Read the model definition and answer for the solid it produces. Units are mm, in the model's axes. A direction names the side the tool comes from. Coordinates: 2 decimals unless noted, no trailing zeros. Answer as a JSON object with one key per item and string values. Group by question number.
1) Which of the six approach directions +Z, -Z, +X, -X, +Y, -Y give full straight-line access (tool end or side, diameter ignored) to faces 1 (the face through (-95, -165, -10)), 2 (the face through (-98.068, -167.218, -0.14))?
2) Consider probe 1 along Y at (x, z) = (70, -0.75); probe 2 along Z at (x, y) = (-253, -156.5); probe 3 along Z at (x, y) = (-36, -130). Determine where each line is inside the solid, lowest interval first. Write a range as [from, to].
3) Flat-ended cylindrical pins translate along their axes: P1, Ø1, axis at y = -81.5, z = -0.5, coming from the -X side; P2, Ø10, axis at y = -115.5, z = -2.5, coming from the +X side; P3, Ø3, axis at x = -90.5, z = -2.5, coming from the -Y side. Find the tip coordinate at first contact, or state that the pin passes through.
from build123d import *

# Parameters (mm, degrees)
ESQUISSE4_R             = 1.5
ESQUISSE6_R             = 3
BOSS_EXTRU_1_DEPTH      = 10
ESQUISSE7_R             = 2
ENL_V_MAT_EXTRU_1_DEPTH = 339.993691721


with BuildPart() as part:
    # Balayage1: sweep along a path in Esquisse3
    with BuildLine(Plane.XY) as balayage1_path:
        Line((-291.161591592, -154.331808471), (-97.417301145, -164.289213701))
        Line((-97.417301145, -164.289213701), (71, -68))
    # Esquisse4 → Balayage1 (sweep)
    with BuildSketch(Plane(origin=(-291.161591592, -154.331808471, 0), x_dir=(-0.05132683108289724, -0.9986819095242427, 0), z_dir=(0.9986819095242427, -0.05132683108289724, 0))):
        Circle(ESQUISSE4_R)
    sweep(path=balayage1_path.line, transition=Transition.RIGHT)

    # Esquisse5 → Révolution1 (revolve)
    with BuildSketch(Plane.XY):
        with BuildLine():
            Line((-288.165545864, -154.485788964), (-294.157637321, -154.177827978))
            ThreePointArc((-294.157637321, -154.177827978), (-291.007611099, -151.335762742), (-288.165545864, -154.485788964))
        make_face()
    revolve(axis=Axis((-288.165545864, -154.485788964, 0), (-0.9986819095242425, 0.05132683108290165, 0)))

    # Esquisse6 → Boss.-Extru.1 (add, symmetric)
    with BuildSketch(Plane.XY):
        with Locations((-97.417301145, -164.289213701)):
            Circle(ESQUISSE6_R)
        with Locations((70, -68)):
            Circle(ESQUISSE6_R)
    extrude(amount=BOSS_EXTRU_1_DEPTH, both=True)

    # Esquisse7 → Enlèv. mat.-Extru.1 (cut, through all)
    with BuildSketch(Plane.XY.offset(10)):
        with Locations((-97.417301145, -164.289213701)):
            Circle(ESQUISSE7_R)
        with Locations((70, -68)):
            Circle(ESQUISSE7_R)
    extrude(amount=-ENL_V_MAT_EXTRU_1_DEPTH, mode=Mode.SUBTRACT)


solid = part.part
Determined:
{
 "1": {"face 1": "-Z, +X, -X, +Y, -Y", "face 2": "none"},
 "2": {"probe 1": "[-71, -70], [-66, -65]", "probe 2": "[-1.49, 1.49]", "probe 3": "[-1.32, 1.32]"},
 "3": {"P1": "x = 43.61", "P2": "x = -1.22", "P3": "y = -161.82"}
}
